```python
from build123d import *

# Parameters (mm, degrees)
F0_W     = 31.305283
F0_H     = 29.811561
F0_H_2   = 38.264022
F0_W_2   = 39.995074
F0_W_3   = 31.305284
F1_DEPTH = 345


with BuildPart() as f1:
    # F0 (on Front) → F1 (new body)
    with BuildSketch(Plane.XZ):
        with Locations((-37.930622, -37.864193)):
            Rectangle(F0_W, F0_H)
        with Locations((-37.930622, -3.826402)):
            Rectangle(F0_W, F0_H_2)
        with Locations((-2.280444, -3.826402)):
            Rectangle(F0_W_2, F0_H_2)
        with Locations((33.369735, -3.826402)):
            Rectangle(F0_W_3, F0_H_2)
        with Locations((33.369735, -37.864193)):
            Rectangle(F0_W_3, F0_H)
    extrude(amount=F1_DEPTH)


solid = f1.part
```
Source: CAD feature listing. Evaluate the final solid. Frame: model axes, mm. A direction names the side the tool comes from. Round coordinates to 2 decimals unless told otherwise and drop trailing zeros. Loops run counter-clockwise (first coordinate to the right, second up) from the corner with the lowest first, then second, coordinate; pieces in that order, holes last.
(1) Access query for faces 1 (the flat face through (33, -170, -52.77)), 2 (the flat face through (17.717, -170, -38)). Directions: +Z, -Z, +X, -X, +Y, -Y. A direction counts if a zero-diameter tool reaches every point of the face in a straight line with its end or side. Return the directions, or none.
From the geometry:
face 1: -Z, +X, -X, +Y, -Y
face 2: -Z, +Y, -Y
(2) Section query B-B (y = -276). Output: boundary loops of the cut face in (x, z).
From the geometry:
outline: (-53.58, -52.77) - (-22.28, -52.77) - (-22.28, -22.96) - (17.72, -22.96) - (17.72, -52.77) - (49.02, -52.77) - (49.02, 15.31) - (-53.58, 15.31) - close
(3) Pull-direction query (X, two-part tool) for faces 3 (the flat face through (-3, 0, -18)), 4 (the flat face through (-22.278, -170, -38)), 5 (the flat face through (49.022, -170, -19)), 6 (the flat face through (-3, -170, -22.958)); classes: +X half, -X half, draft (parallel to the pull), parting line (faces both ways), or undercut.
From the geometry:
face 3: draft
face 4: undercut
face 5: +X half
face 6: undercut
(4) Section query C-C (x = 3.5). Output: boundary loops of the cut face in (y, z), and give its area (3 significant figures).
From the geometry:
outline: (-345, -22.96) - (0, -22.96) - (0, 15.31) - (-345, 15.31) - close
area: 13,200 mm2
(5) Material intervals for probe 1 along X at (y, z) = (-157.5, -28.5); probe 2 along Z at (x, y) = (-7.5, -73.5), sorted ascending.
From the geometry:
probe 1: x = -53.58 to -22.28, 17.72 to 49.02
probe 2: z = -22.96 to 15.31
(6) Contact query for flat-ended pins moving along their axis: pin 1 Ø6 at (x, y) = (-22, -285.5) entering from -Z; pin 2 Ø6 at (x, y) = (14.5, -277) entering from -Z. Output: stop coordinate, or through.
From the geometry:
pin 1: stops at z = -52.77
pin 2: stops at z = -22.96
(7) Section query A-A (z = -46). Output: boundary loops of the cut face in (x, y), and give its area (3 significant figures).
From the geometry:
outline: (-53.58, -345) - (-22.28, -345) - (-22.28, 0) - (-53.58, 0) - close; (17.72, -345) - (49.02, -345) - (49.02, 0) - (17.72, 0) - close
area: 21,600 mm2
